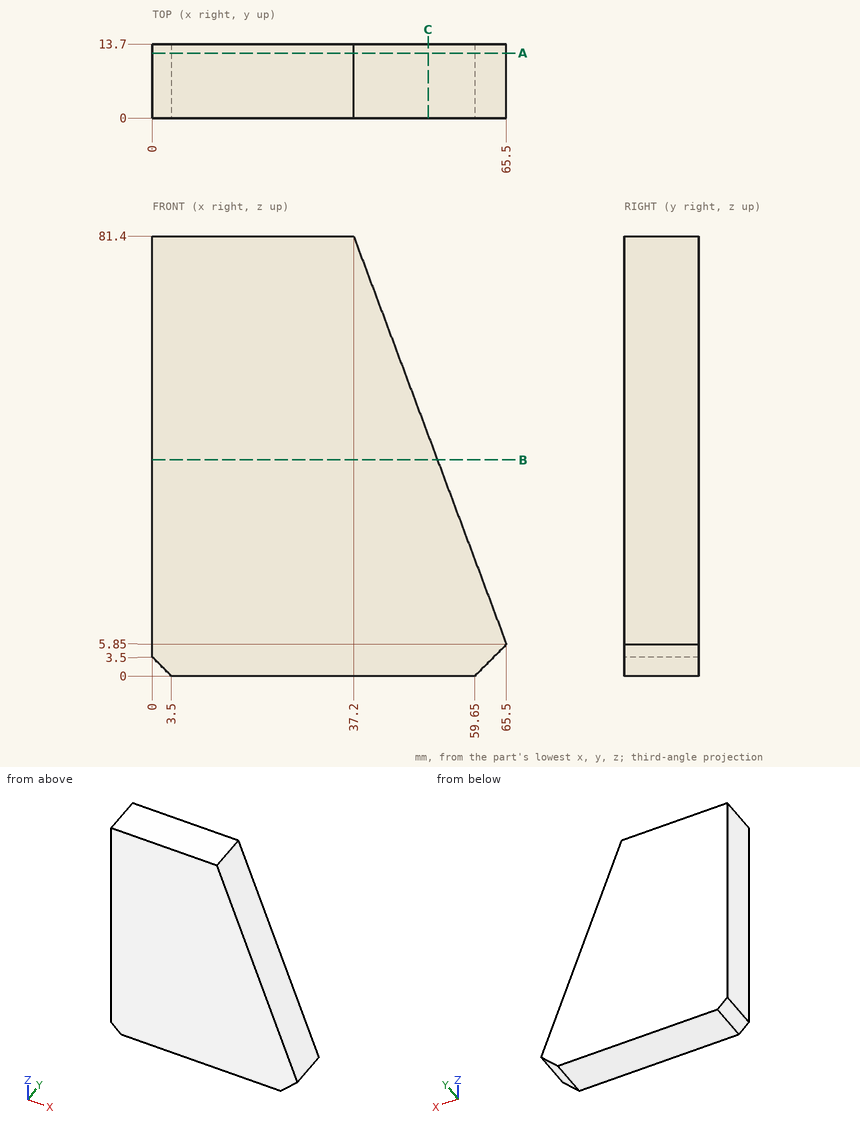
Study the drawing (mm; zero at the part's minimum x, y, z) and answer. Round coordinates to 2 decimals unless told otherwise and drop trailing zeros. Write each loop counter-clockwise with the first axis right and the second up, starting at its lowest first coordinate (ties: lowest second). Pieces come first, ordered by that corner, then holes.
1) Straight lines are drawn through the part: line 1 (X direction, y = 5, z = 77); line 2 (X direction, y = 2, z = 21.5). For each, find the intervals that lie inside material, in ascending order.
2) A cutting plane is placed at C-C (x = 51). Give the vertices of the cut face in (y, z), plus the area to 3 significant figures.
3) A cutting plane is placed at A-A (y = 12). Give the vertices of the cut face in (x, z), plus the area to 3 significant figures.
4) Given pin 1 Ø3 at (x, y) = (34.5, 3.5) entering from -Z, flat-ended and moving along its own axis, determine where the tip first touches the part or whether it passes through.
5) A cutting plane is placed at B-B (z = 40). Give the vertices of the cut face in (x, y).
Completed:
1. line 1: x = 0 to 38.85
1. line 2: x = 0 to 59.64
2. outline: (0, 0) - (13.7, 0) - (13.7, 44.56) - (0, 44.56) - close
2. area: 610 mm2
3. outline: (0, 3.5) - (3.5, 0) - (59.65, 0) - (65.5, 5.85) - (37.2, 81.4) - (0, 81.4) - close
3. area: 4,240 mm2
4. pin 1: stops at z = 0
5. outline: (0, 0) - (52.71, 0) - (52.71, 13.7) - (0, 13.7) - close
